Autodesk Inventor part; units mm, degrees
ref_plane "YZ Plane" through (0, 0, 0) normal (1, 0, 0) x (0, 1, 0)
ref_plane "XZ Plane" through (0, 0, 0) normal (0, 1, 0) x (-1, 0, 0)
ref_plane "XY Plane" through (0, 0, 0) normal (0, 0, 1) x (1, 0, 0)
sketch "Sketch1" plane through (0, 0, 0) normal (0, 0, 1) x (1, 0, 0)
  circle A0 centre (0, 0) radius 34.925
  dimension "d0" = 69.85
extrude "Extrusion1" add sketch "Sketch1" along normal blind 2.54
sketch "Sketch2" plane through (0, 0, 2.54) normal (0, 0, 1) x (1, 0, 0)
  circle A0 centre (0, 0) radius 11.1125
  line L0 (0, 0) -> (0, -12.7)
  circle A1 centre (0, -12.7) radius 4.7625
  circle A2 centre (10.9985, 6.35) radius 4.7625
  circle A3 centre (-10.9985, 6.35) radius 4.7625
  dimension "d3" = 22.225
  dimension "d4" = 12.7
  dimension "d5" = 9.525
  dimension "d8" = 360
extrude "Extrusion2" add sketch "Sketch2" along normal blind 6.35 contours A0 A1 A3 A2 | A2 A0 | A0 L0 A1 | A0 A1 L0 | A3 A0 picked at (9.3538, 3.9651) picked at (-8.1265, 6.0404)
extrude "Extrusion3" cut sketch "Sketch2" along normal blind 6.35 contours A2 A0 | A0 A2 | A1 A0 | A0 L0 A1 | A0 A1 L0 | A3 A0 | A0 A3
sketch "Sketch3" plane through (0, 0, 2.54) normal (0, 0, 1) x (1, 0, 0)
  line L0 (0, 0) -> (0, 9.525)
  circle A0 centre (0, 9.525) radius 3.175
  dimension "d14" = 9.525
  dimension "d15" = 6.35
extrude "Extrusion4" add sketch "Sketch3" along normal blind 6.35
sketch "Sketch4" plane through (0, 0, 8.89) normal (0, 0, 1) x (1, 0, 0)
  circle A0 centre (0, 0) radius 3.175
  circle A1 centre (0, 0) radius 2.3813
  dimension "d18" = 6.35
  dimension "d19" = 4.7625
extrude "Extrusion5" cut sketch "Sketch4" against normal blind 3.175 contours A0 | A1
extrude "Extrusion6" cut sketch "Sketch4" against normal through all contours A1
properties part number "SpoolEndSpurSide" material "ABS Plastic"
Check sheet for the modelled part. Datum: model origin and axes. Units: mm. A direction names the side the tool comes from. Round coordinates to 2 decimals unless told otherwise and drop trailing zeros. Loops run counter-clockwise (first coordinate to the right, second up) from the corner with the lowest first, then second, coordinate; pieces in that order, holes last. Notation, with made-up numbers: M 43,48 L 100,48 A22 cw 100,55 Z; hole C 73,-8 d1. An arc over 180 degrees is marked long. One line per question, with ' | ' between items. Start each with the question number.
Item 1: Section check C-C (y = 0). Record the boundary of the cut face in (x, z) (1 decimal).
Item 2: Release check for a two-part mould opening along Y. For faces 1 (the face through (-0.69, -3.1, 7.32)), 2 (the face through (-0.07, -7.94, 5.67)), 3 (the face through (0, 4, 8.89)), 4 (the face through (-0.1, 12.7, 5.7)) record: released by +Y, released by -Y, zero draft, split by the parting line, or undercut.
Item 3: Section check A-A (x = 0). Record the boundary of the cut face in (y, z) (1 decimal).
Item 4: Set-up check for faces 5 (the face through (7, 8, 2.54)), 6 (the face through (-6.84, 4.03, 5.67)), 7 (the face through (6.91, 3.91, 5.67)), 8 (the face through (-5.036, 9.906, 5.671)): record each of +Z, -Z, +X, -X, +Y, -Y from which the full face is reachable in a straight line by a thin tool's end or side.
Item 5: Gauge pin test, flat ends, axial feed: pin 1 Ø1 at (x, z) = (6, 3.5) entering from +Y; pin 2 Ø6 at (x, y) = (-3.5, -20) entering from +Z; pin 3 Ø5.5 at (x, y) = (0, 0) entering from +Z (3 decimals). Record the tip position at first contact, or that the pin passes through.
Item 6: Scan lines: probe 1 along Y at (x, z) = (0, 1.8) (3 decimals); probe 2 along Z at (x, y) = (27.5, -9); probe 3 along X at (y, z) = (4, 3). Record each from-to range of solid material in increasing order.
Item 7: Section check D-D (x = 8). Record the boundary of the cut face in (y, z), and give its area (3 significant figures).
Worked out:
1) outline: M -34.9,0 L -2.4,0 L -2.4,5.7 L -3.2,5.7 L -3.2,8.9 L -11.1,8.9 L -11.1,2.5 L -34.9,2.5 Z; M 2.4,0 L 34.9,0 L 34.9,2.5 L 11.1,2.5 L 11.1,8.9 L 3.2,8.9 L 3.2,5.7 L 2.4,5.7 Z
2) face 1: undercut | face 2: released by -Y | face 3: zero draft | face 4: released by +Y
3) outline: M -34.9,0 L -2.4,0 L -2.4,5.7 L -3.2,5.7 L -3.2,8.9 L -7.9,8.9 L -7.9,2.5 L -34.9,2.5 Z; M 2.4,0 L 34.9,0 L 34.9,2.5 L 12.7,2.5 L 12.7,8.9 L 3.2,8.9 L 3.2,5.7 L 2.4,5.7 Z
4) face 5: +Z | face 6: +Z, -X | face 7: +Z, +X | face 8: +Z, -X, +Y
5) pin 1: y = 9.66 | pin 2: z = 2.54 | pin 3: z = 5.715
6) probe 1: -34.925 to -2.381, 2.381 to 34.925 | probe 2: 0 to 2.54 | probe 3: -6.86 to 6.86
7) outline: M -34,0 L 34,0 L 34,2.54 L 2.65,2.54 L 2.65,8.89 L -7.71,8.89 L -7.71,2.54 L -34,2.54 Z | area: 239 mm^2
